Source: three-view drawing plus pictorial views. Frame: mm from the lowest corner of the part. A direction names the side the tool comes from. Round coordinates to 2 decimals unless told otherwise and drop trailing zeros. Loops run counter-clockwise (first coordinate to the right, second up) from the corner with the lowest first, then second, coordinate; pieces in that order, holes last. Notation, with made-up numbers: (-13, 89) -> (-1, 89) arc R26 ccw to (-1, 115) -> close; hole circle Ø3 at (48, 52.25). An arc over 180 degrees is marked (long way). Answer in a Markdown table with one row per item. Add a question column.
Q1. Mould query, pull axis Z, two halves, no side actions, for the marked faces 1, 2, 3 and 4. Classes: pulls with the +Z half, pulls with the -Z half, needs draft (parallel to the pull), parting line crosses it, or undercut.
Q2. Section A-A, the plane y = 10.5. Output: boundary loops of the cut face in (x, z).
Q3. Section D-D, the plane z = 6.5. Output: boundary loops of the cut face in (x, y), and give its area (4 significant figures).
Q4. Pin query (flat end, axial travel): pin 1 (3 mm diameter, centred on x = 4.5, y = 9, fed in from -Z); pin 2 (1 mm diameter, centred on x = 2.5, z = 13.5, fed in from -Y); pin 3 (2 mm diameter, centred on x = 4.5, z = 4.5, fed in from +Y). Return the tip coordinate at first contact, or that it passes through.
Q5. Section B-B, the plane x = 0.75. Output: boundary loops of the cut face in (y, z), and give its area (4 significant figures).
Q6. Reachability of the marked faces 5, 6, 7 and 8 from +Z, -Z, +X, -X, +Y, -Y: full face, straight path, thin tool, end or side. Return the list, or none.
Q7. Section C-C, the plane z = 12. Output: boundary loops of the cut face in (x, y).
Q8. Ray query, L1, parallel to Z at x = 2.25, y = 12.75; L2, parallel to X at y = 1.5, z = 15; L3, parallel to Y at x = 4.5, z = 17.5. Return the intervals inside material, ascending. Write a range as from..to.
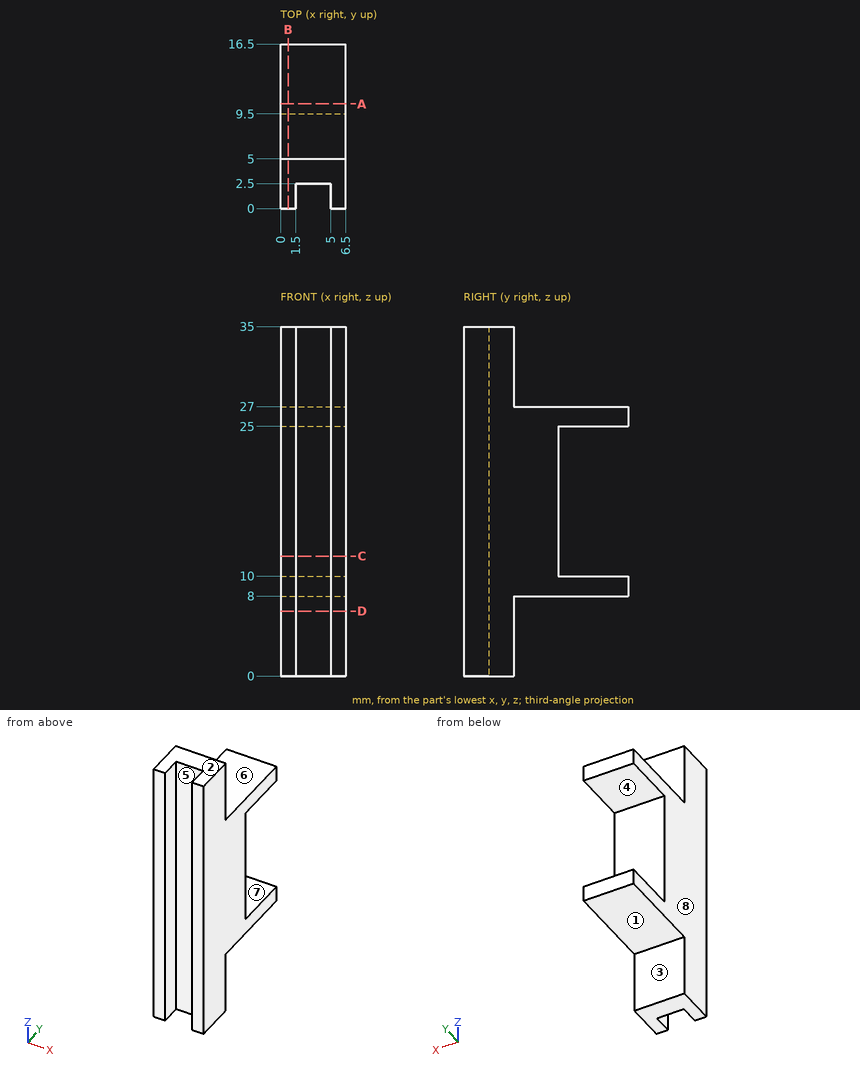
Answer block:
| question | item | result |
|---|---|---|
| 1 | face 1 | pulls with the -Z half |
| 1 | face 2 | pulls with the +Z half |
| 1 | face 3 | needs draft |
| 1 | face 4 | undercut |
| 2 | outline | (0, 8) -> (6.5, 8) -> (6.5, 10) -> (0, 10) -> close; (0, 25) -> (6.5, 25) -> (6.5, 27) -> (0, 27) -> close |
| 3 | outline | (0, 0) -> (1.5, 0) -> (1.5, 2.5) -> (5, 2.5) -> (5, 0) -> (6.5, 0) -> (6.5, 5) -> (0, 5) -> close |
| 3 | area | 23.75 mm^2 |
| 4 | pin 1 | z = 8 |
| 4 | pin 2 | y = 2.5 |
| 4 | pin 3 | y = 5 |
| 5 | outline | (0, 0) -> (5, 0) -> (5, 8) -> (16.5, 8) -> (16.5, 10) -> (9.5, 10) -> (9.5, 25) -> (16.5, 25) -> (16.5, 27) -> (5, 27) -> (5, 35) -> (0, 35) -> close |
| 5 | area | 288.5 mm^2 |
| 6 | face 5 | +Z, -Z, -Y |
| 6 | face 6 | +Z, +X, -X, +Y |
| 6 | face 7 | +X, -X, +Y |
| 6 | face 8 | +Z, -Z, -X, +Y, -Y |
| 7 | outline | (0, 0) -> (1.5, 0) -> (1.5, 2.5) -> (5, 2.5) -> (5, 0) -> (6.5, 0) -> (6.5, 9.5) -> (0, 9.5) -> close |
| 8 | L1 | 8..10, 25..27 |
| 8 | L2 | 0..1.5, 5..6.5 |
| 8 | L3 | 2.5..9.5 |
